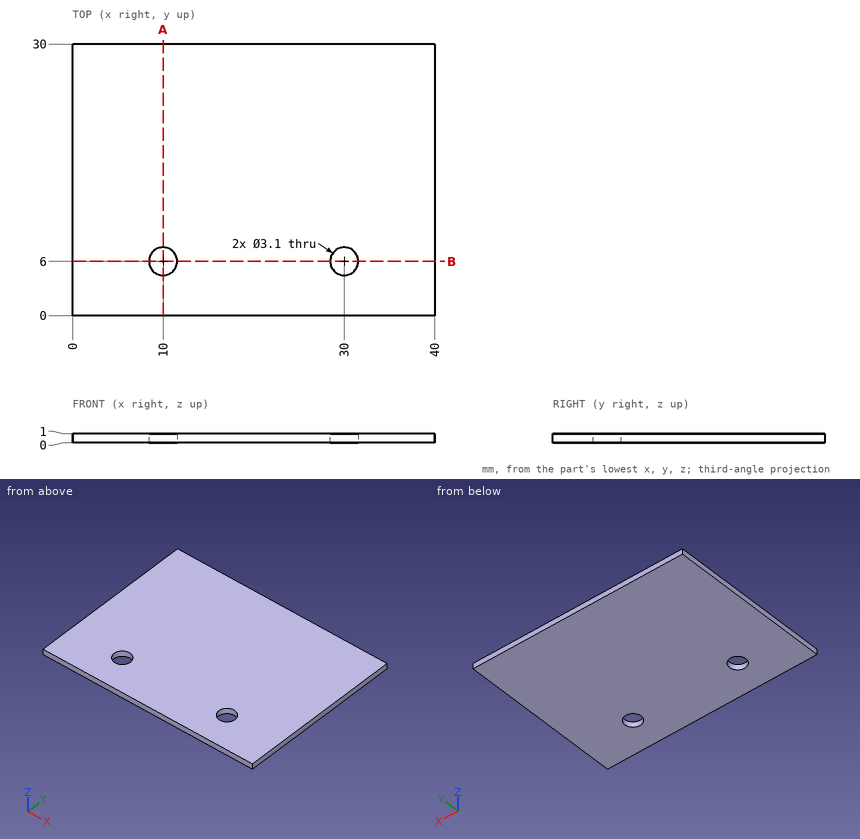
Verification items for this drawing (mm, ordinates from the low corner). Coordinates: 2 decimals unless noted, no trailing zeros. Order: outer loops, then holes, each group sorted by start corner. A loop starts at its lowest first (then second) coordinate and runs counter-clockwise, first axis right, second up.
Q1. Thickness scan on probe 1 along Y at (x, z) = (30, 0.2); probe 2 along X at (y, z) = (4.75, 0.15); probe 3 along X at (y, z) = (7, 0.5). Record the ranges inside material, lowest first.
Reply:
probe 1: y = 0 to 4.45, 7.55 to 30
probe 2: x = 0 to 9.08, 10.92 to 29.08, 30.92 to 40
probe 3: x = 0 to 8.82, 11.18 to 28.82, 31.18 to 40
Q2. Sectioned sample at B-B on y = 6. Record the cut outline in (x, z), and give its area (3 significant figures).
Reply:
outline: (0, 0) - (8.45, 0) - (8.45, 1) - (0, 1) - close; (11.55, 0) - (28.45, 0) - (28.45, 1) - (11.55, 1) - close; (31.55, 0) - (40, 0) - (40, 1) - (31.55, 1) - close
area: 33.8 mm2
Q3. Sectioned sample at A-A on x = 10. Record the cut outline in (y, z).
Reply:
outline: (0, 0) - (4.45, 0) - (4.45, 1) - (0, 1) - close; (7.55, 0) - (30, 0) - (30, 1) - (7.55, 1) - close
